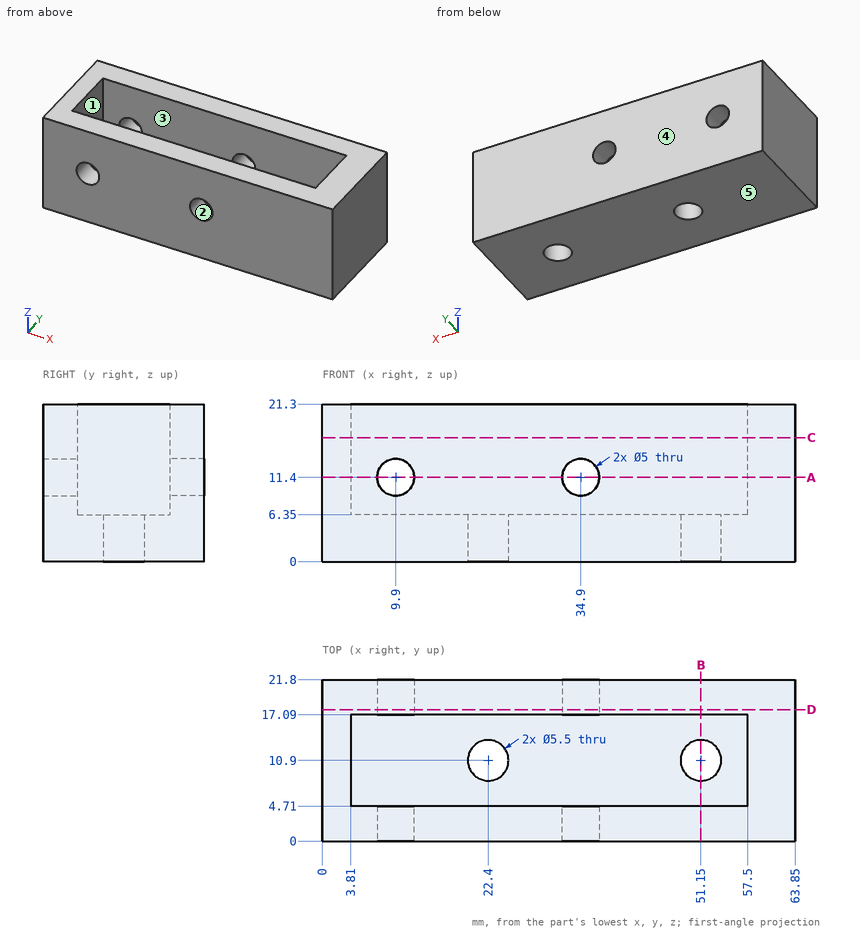
Source: three-view drawing plus pictorial views. Frame: mm from the lowest corner of the part. A direction names the side the tool comes from. Round coordinates to 2 decimals unless told otherwise and drop trailing zeros. Loops run counter-clockwise (first coordinate to the right, second up) from the corner with the lowest first, then second, coordinate; pieces in that order, holes last.
1. Contact query for flat-ended pins moving along their axis: pin 1 (10 mm diameter, centred on y = 16, z = 3.5, fed in from -X); pin 2 (9 mm diameter, centred on x = 22.4, y = 10.9, fed in from +Z). Output: stop coordinate, or through.
2. Access query for the marked faces 1 and 2. Directions: +Z, -Z, +X, -X, +Y, -Y. A direction counts if a zero-diameter tool reaches every point of the face in a straight line with its end or side. Return the directions, or none.
3. Section query C-C on z = 16.75. Output: boundary loops of the cut face in (x, y), and give its area (3 significant figures).
4. Section query B-B on x = 51.15. Output: boundary loops of the cut face in (y, z).
5. Ray query, L1, parallel to X at y = 20.2, z = 11.4; L2, parallel to Y at x = 22, z = 9.5; L3, parallel to Y at x = 51.15, z = 5.25. Return the intervals inside material, ascending.
6. Section query D-D on y = 17.75. Output: boundary loops of the cut face in (x, z).
7. Mould query, pull axis Y, two halves, no side actions, for the marked faces 3, 4 and 5. Classes: released by +Y, released by -Y, zero draft, split by the parting line, or undercut.
8. Section query A-A on z = 11.4. Output: boundary loops of the cut face in (x, y).
Answers below:
1. pin 1: stops at x = 0
1. pin 2: stops at z = 6.35
2. face 1: +Z
2. face 2: +Y, -Y
3. outline: (0, 0) - (63.85, 0) - (63.85, 21.8) - (0, 21.8) - close; hole (3.81, 4.71) - (57.5, 4.71) - (57.5, 17.09) - (3.81, 17.09) - close
3. area: 727 mm2
4. outline: (0, 0) - (8.15, 0) - (8.15, 6.35) - (4.71, 6.35) - (4.71, 21.3) - (0, 21.3) - close; (13.65, 0) - (21.8, 0) - (21.8, 21.3) - (17.09, 21.3) - (17.09, 6.35) - (13.65, 6.35) - close
5. L1: x = 0 to 7.4, 12.4 to 32.4, 37.4 to 63.85
5. L2: y = 0 to 4.71, 17.09 to 21.8
5. L3: y = 0 to 8.15, 13.65 to 21.8
6. outline: (0, 0) - (63.85, 0) - (63.85, 21.3) - (0, 21.3) - close; hole circle Ø5 at (9.9, 11.4); hole circle Ø5 at (34.9, 11.4)
7. face 3: undercut
7. face 4: released by +Y
7. face 5: zero draft
8. outline: (0, 0) - (7.4, 0) - (7.4, 4.71) - (3.81, 4.71) - (3.81, 17.09) - (7.4, 17.09) - (7.4, 21.8) - (0, 21.8) - close; (12.4, 0) - (32.4, 0) - (32.4, 4.71) - (12.4, 4.71) - close; (12.4, 17.09) - (32.4, 17.09) - (32.4, 21.8) - (12.4, 21.8) - close; (37.4, 0) - (63.85, 0) - (63.85, 21.8) - (37.4, 21.8) - (37.4, 17.09) - (57.5, 17.09) - (57.5, 4.71) - (37.4, 4.71) - close
